from build123d import *

# Parameters (mm, degrees)
F0_W     = 19.65
F0_H     = 1.5
F1_DEPTH = 1


# Not quite as in the source:
# - a feature names something its author has since deleted; it is built from what else it names


with BuildPart() as f1:
    # F0 (on Right) → F1 (new body)
    with BuildSketch(Plane.YZ):
        Polygon((121.65, -16.375), (19.65, -16.375), (-19.65, -16.375), (-61.65, -16.375), (-61.65, -39.125), (121.65, -39.125), align=None)
        Polygon((-19.65, -16.375), (19.65, -16.375), (19.65, 14.875), (0, 14.875), (-19.65, 14.875), align=None)
        Polygon((19.65, 14.875), (19.65, -16.375), (121.65, -16.375), (121.65, 16.375), (19.65, 16.375), align=None)
        Polygon((-61.65, -16.375), (-19.65, -16.375), (-19.65, 14.875), (-19.65, 16.375), (-19.65, 57.475), (-19.65, 92.575), (-121.65, 92.575), (-121.65, 89.375), (-121.65, 16.375), (-111.65, 16.375), (-75.65, 16.375), (-61.65, 16.375), align=None)
        with Locations((9.825, 15.625)):
            Rectangle(F0_W, F0_H)
        with Locations((-9.825, 15.625)):
            Rectangle(F0_W, F0_H)
        with BuildLine():
            Line((-61.65, -39.125), (-61.65, -16.375))
            Line((-61.65, -16.375), (-121.65, -16.375))
            Line((-121.65, -16.375), (-121.65, -39.125))
            Line((-121.65, -39.125), (-111.65, -39.125))
            ThreePointArc((-111.65, -39.125), (-92.65, -20.125), (-73.65, -39.125))
            Line((-73.65, -39.125), (-61.65, -39.125))
        make_face()
        Polygon((-121.65, -16.375), (-61.65, -16.375), (-61.65, 16.375), (-75.65, 16.375), (-111.65, 16.375), (-121.65, 16.375), align=None)
        with BuildLine():
            ThreePointArc((-108.65, 8.375), (-113.7713203436, 6.2536796564), (-111.65, 11.375))
            ThreePointArc((-111.65, 11.375), (-109.5286796564, 10.4963203436), (-108.65, 8.375))
        make_face(mode=Mode.SUBTRACT)
        with BuildLine():
            ThreePointArc((-72.65, 8.375), (-77.7713203436, 6.2536796564), (-75.65, 11.375))
            ThreePointArc((-75.65, 11.375), (-73.5286796564, 10.4963203436), (-72.65, 8.375))
        make_face(mode=Mode.SUBTRACT)
        Polygon((19.65, 57.475), (19.65, 16.375), (121.65, 16.375), (121.65, 89.375), (121.65, 92.575), (19.65, 92.575), align=None)
        Polygon((0, 16.375), (19.65, 16.375), (19.65, 57.475), (6, 57.475), (6, 29.475), (0, 29.475), align=None)
        Polygon((-19.65, 57.475), (-19.65, 16.375), (0, 16.375), (0, 29.475), (-6, 29.475), (-6, 57.475), align=None)
        Polygon((6, 57.475), (19.65, 57.475), (19.65, 92.575), (18, 92.575), (18, 105.675), (18, 107.675), (17, 107.675), (17, 132.675), (18, 132.675), (0, 150.675), (0, 132.675), (13, 132.675), (13, 105.675), (0, 105.675), (0, 93.575), (6, 93.575), (6, 92.575), (6, 89.375), (6, 70.575), (6, 68.575), align=None)
        Polygon((-19.65, 92.575), (-19.65, 57.475), (-6, 57.475), (-6, 29.475), (0, 29.475), (6, 29.475), (6, 57.475), (6, 68.575), (-6, 68.575), (-6, 70.575), (-6, 92.575), (-6, 93.575), (0, 93.575), (0, 105.675), (-13, 105.675), (-13, 132.675), (0, 132.675), (0, 150.675), (-18, 132.675), (-17, 132.675), (-17, 107.675), (-18, 107.675), (-18, 105.675), (-18, 92.575), align=None)
        with BuildLine():
            Line((-77.15, -39.125), (-73.65, -39.125))
            ThreePointArc((-73.65, -39.125), (-92.65, -20.125), (-111.65, -39.125))
            Line((-111.65, -39.125), (-108.15, -39.125))
            ThreePointArc((-108.15, -39.125), (-92.65, -23.625), (-77.15, -39.125))
        make_face()
    extrude(amount=F1_DEPTH)


solid = f1.part
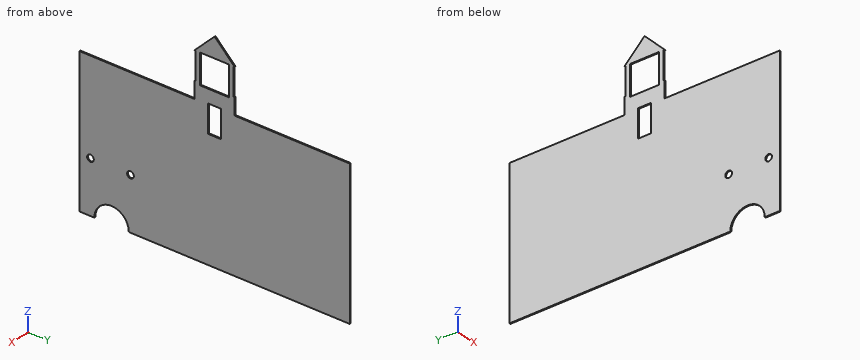
Work out the finished part from the listing and answer in its coordinate system (mm). Give positions to 0.01 mm unless a question says otherwise; leave off trailing zeros. Order: outer loops, then holes, each group sorted by start corner. A loop starts at its lowest first (then second) coordinate and runs counter-clockwise, first axis right, second up. Notation, with made-up numbers: M 67,-32 L 85,-32 A15 ccw 85,-16 Z; hole C 7.5,36 d2. An arc over 180 degrees is marked long. Return JSON: item names as keys, results as strings.
Q1. Find section A-A, the plane x = 0.5. Write down the section's boundary in (y, z) (3 decimals), and give its area (3 significant figures).
Answer below:
{"outline": "M -121.65,-39.125 L -108.15,-39.125 A15.5 cw -77.15,-39.125 L 121.65,-39.125 L 121.65,92.575 L 18,92.575 L 18,107.675 L 17,107.675 L 17,132.675 L 18,132.675 L 0,150.675 L -18,132.675 L -17,132.675 L -17,107.675 L -18,107.675 L -18,92.575 L -121.65,92.575 Z; hole C -111.65,8.375 d6; hole C -75.65,8.375 d6; hole M -13,105.675 L 13,105.675 L 13,132.675 L -13,132.675 Z; hole M -6,68.575 L 6,68.575 L 6,93.575 L -6,93.575 Z", "area": "32,300 mm^2"}
Q2. Find section D-D, the plane y = -92.65. Write down the section's boundary in (x, z) (3 decimals), and give its area (3 significant figures).
Answer below:
{"outline": "M 0,-23.625 L 1,-23.625 L 1,92.575 L 0,92.575 Z", "area": "116 mm^2"}
Q3. This flat-tipped pin is pushed along its axis until it touches: pin 1 (0.5 mm diameter, centred on x = 0.5, z = 124, fed in from +Y). Where does it stop, or does it pass through?
Answer below:
{"pin 1": "stops at y = 17"}
Q4. Find section B-B, the plane z = 124.5. Write down the section's boundary in (x, y).
Answer below:
{"outline": "M 0,-17 L 1,-17 L 1,-13 L 0,-13 Z; M 0,13 L 1,13 L 1,17 L 0,17 Z"}
Q5. Find section C-C, the plane z = 82.5. Write down the section's boundary in (x, y), and give its area (3 significant figures).
Answer below:
{"outline": "M 0,-121.65 L 1,-121.65 L 1,-6 L 0,-6 Z; M 0,6 L 1,6 L 1,121.65 L 0,121.65 Z", "area": "231 mm^2"}
Q6. Find the intervals of material crossed by line 1 along Y through (x, z) = (0.6, 75); line 2 along Y through (x, z) = (0.65, 115.5); line 3 along Z through (x, y) = (0.55, -111.65) (3 decimals), in increasing order. Write a range as [from, to].
Answer below:
{"line 1": "y = [-121.65, -6], [6, 121.65]", "line 2": "y = [-17, -13], [13, 17]", "line 3": "z = [-39.125, 5.375], [11.375, 92.575]"}
